Answer from the drawing. Dimensions are ordinates in mm from the lowest x, y and z of the part. Coordinates: 2 decimals unless noted, no trailing zeros. Write each loop counter-clockwise with the first axis right and the second up, starting at its lowest first coordinate (ties: lowest second). Pieces come first, ordered by that corner, then holes.
(1) Given pin 1 (8 mm diameter, centred on x = 32, y = 3.5, fed in from -Z); pin 2 (2 mm diameter, centred on x = 17.5, y = 9, fed in from +Z), each flat-ended and moving along its own axis, determine where each tip first touches the part or whether it passes through.
(2) Straight lines are drawn through the part: line 1 along X through (y, z) = (6, 0.3); line 2 along Y through (x, z) = (6, 0.6); line 3 along X through (y, z) = (5.75, 0.3). For each, find the intervals that lie inside material, in ascending order.
(3) The part is cut by section D-D, the plane x = 20. Determine the outline of the cut face in (y, z).
(4) The part is cut by section A-A, the plane x = 9. Determine the outline of the cut face in (y, z).
(5) The part is cut by section C-C, the plane z = 0.8. Determine the outline of the cut face in (x, y).
(6) The part is cut by section B-B, the plane y = 9. State how many separate pieces and enclosed holes the cut face has.
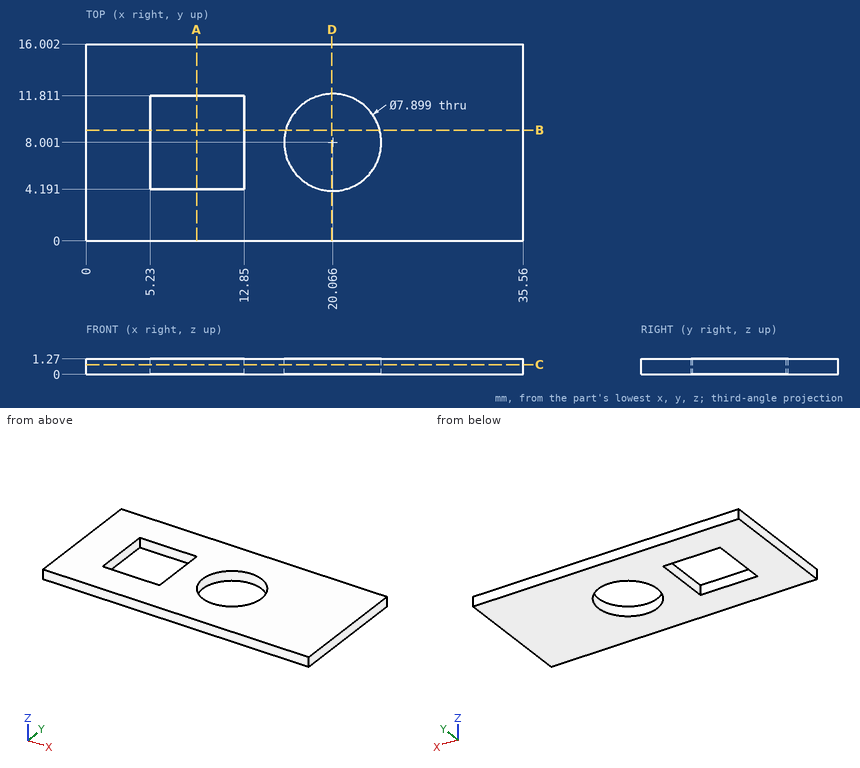
Computed:
1. pin 1: stops at z = 0
1. pin 2: passes through
2. line 1: x = 0 to 5.23, 12.85 to 16.66, 23.47 to 35.56
2. line 2: y = 0 to 4.19, 11.81 to 16
2. line 3: x = 0 to 5.23, 12.85 to 16.82, 23.31 to 35.56
3. outline: (0, 0) - (4.05, 0) - (4.05, 1.27) - (0, 1.27) - close; (11.95, 0) - (16, 0) - (16, 1.27) - (11.95, 1.27) - close
4. outline: (0, 0) - (4.19, 0) - (4.19, 1.27) - (0, 1.27) - close; (11.81, 0) - (16, 0) - (16, 1.27) - (11.81, 1.27) - close
5. outline: (0, 0) - (35.56, 0) - (35.56, 16) - (0, 16) - close; hole (5.23, 4.19) - (12.85, 4.19) - (12.85, 11.81) - (5.23, 11.81) - close; hole circle Ø7.9 at (20.07, 8)
6. separate pieces: 3
6. enclosed holes: 0
